Work out the finished part from the listing and answer in its coordinate system (mm). Face numbers are marked on the shaded views. Coordinates: 2 decimals unless noted, no trailing zeros. Order: outer loops, then holes, each group sorted by start corner. A loop starts at its lowest first (then second) coordinate and runs counter-clockwise, first axis right, second up. Notation, with made-up numbers: M -7,-29 L 15,-29 A31 cw 15,0 Z; hole C 80,17 d6. An arc over 180 degrees is marked long. Write item = value, one per line. Start each with the question number.
Q1. Find section C-C on y = 22. Give the vertices of the cut face in (x, z).
Q2. Each of these flat-tipped pins is pushed along its axis until it touches: P1, Ø3, axis at x = 4.5, y = 25.5, coming from the -Z side; P2, Ø3, axis at y = -21.5, z = -2, coming from the -X side; P3, Ø6, axis at x = 0, z = 0, coming from the +Y side. Where does it stop, or does it pass through?
Q3. Determine the mould class of the marked faces 1, 2 and 3 for opening direction Z: released by +Z, released by -Z, zero draft, split by the parting line, or undercut.
Q4. Find section D-D on x = 5.75. Give the vertices of the cut face in (y, z), and give its area (3 significant figures).
Q5. Find section A-A on z = 0. Give the vertices of the cut face in (x, y).
Q6. Straight lines are drawn through the part: line 1 along X through (y, z) = (38.8, 0); line 2 along X through (y, z) = (39.1, 0); line 3 along Y through (x, z) = (-3, 5.25). For each, find the intervals that lie inside material, in ascending order.
```python
from build123d import *

# Parameters (mm, degrees)
CROQUIS1_W                          = 7.5
CROQUIS1_H                          = 47.25
CROQUIS2_R                          = 3.2
SALIENTE_EXTRUIR1_DEPTH             = 1
CROQUIS3_R                          = 2.5
SALIENTE_EXTRUIR2_DEPTH             = 23
CORTAR_EXTRUIR1_START               = -20
CORTAR_EXTRUIR1_DEPTH               = 20
DI_METRO_DE_TALADRO_6_4_6_4_1_D     = 6.4
DI_METRO_DE_TALADRO_6_4_6_4_1_DEPTH = 1
CROQUIS7_W                          = 2.5
CROQUIS7_H                          = 0.75
CHAFL_N1_SIZE                       = 0.25


with BuildPart() as part:
    # Croquis1 → Revolución1 (revolve)
    with BuildSketch(Plane(origin=(0, 0, 0), x_dir=(-1, 0, 0), z_dir=(0, 0, -1)), mode=Mode.PRIVATE) as revoluci_n1_sk:
        with Locations((-3.75, 15.625)):
            Rectangle(CROQUIS1_W, CROQUIS1_H)
    revolve(revoluci_n1_sk.sketch.rotate(Axis((0, -8, 0), (0, 1, 0)), 270), axis=Axis((0, -8, 0), (0, 1, 0)))

    # Croquis2 → Saliente-Extruir1 (add)
    with BuildSketch(Plane.XZ.offset(8)):
        with Locations(Location((0, 0, 0), (0, 0, 270))):
            Circle(CROQUIS2_R)
    extrude(amount=SALIENTE_EXTRUIR1_DEPTH)

    # Croquis3 → Saliente-Extruir2 (add)
    with BuildSketch(Plane.XZ.offset(9)):
        with Locations(Location((0, 0, 0), (0, 0, 270))):
            Circle(CROQUIS3_R)
    extrude(amount=SALIENTE_EXTRUIR2_DEPTH)

    # Croquis4 → Cortar-Extruir1 (cut)
    with BuildSketch(Plane.XZ.offset(32).offset(CORTAR_EXTRUIR1_START)):
        with BuildLine():
            Line((-1.356465997, 2.1), (1.356465997, 2.1))
            ThreePointArc((1.356465997, 2.1), (0, 2.5), (-1.356465997, 2.1))
        make_face()
    extrude(amount=CORTAR_EXTRUIR1_DEPTH, mode=Mode.SUBTRACT)

    # Diámetro de taladro Ø6.4 (6.4)1
    with Locations(Plane(origin=(0, 39.25, 0), x_dir=(1, 0, 0), z_dir=(0, 1, 0))):
        with Locations((0, 0)):
            Hole(DI_METRO_DE_TALADRO_6_4_6_4_1_D / 2, depth=DI_METRO_DE_TALADRO_6_4_6_4_1_DEPTH)

    # Croquis7 → Revolución2 (revolve)
    with BuildSketch(Plane(origin=(0, 0, 0), x_dir=(-1, 0, 0), z_dir=(0, 0, -1)), mode=Mode.PRIVATE) as revoluci_n2_sk:
        with Locations((-1.25, 38.625)):
            Rectangle(CROQUIS7_W, CROQUIS7_H)
    revolve(revoluci_n2_sk.sketch.rotate(Axis((0, 38.25, 0), (0, 1, 0)), 270), axis=Axis((0, 38.25, 0), (0, 1, 0)))

    # Chaflán1
    chafl_n1_edges = [part.edges().sort_by_distance(p)[0] for p in [
        (0, -9, 3.2),
        (-2.397915762, -32, -0.707106781),
        (3.2, 38.25, 0),
        (0, 39, -2.5),
    ]]
    chamfer(chafl_n1_edges, length=CHAFL_N1_SIZE)


solid = part.part
```
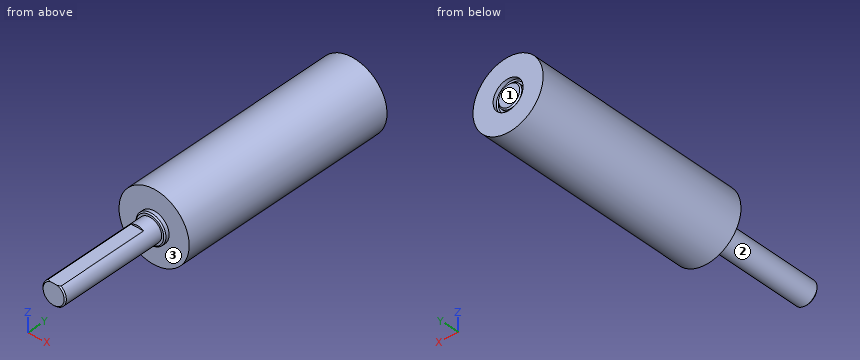
Findings below:
q1.outline = C 0,0 d15
q2.P1 = -6.87
q2.P2 = -2.45
q2.P3 = 39
q3.face_1 = undercut
q3.face_2 = split by the parting line
q3.face_3 = zero draft
q4.outline = M -8,-4.82 L 39.25,-4.82 L 39.25,4.82 L -8,4.82 Z
q4.area = 455 mm^2
q5.outline = M -7.5,-8 L -3.2,-8 L -3.2,-8.75 L -2.95,-9 L -2.5,-9 L -2.5,-31.75 L -2.25,-32 L 2.25,-32 L 2.5,-31.75 L 2.5,-9 L 2.95,-9 L 3.2,-8.75 L 3.2,-8 L 7.5,-8 L 7.5,39.25 L 3.2,39.25 L 3.2,38.5 L 2.95,38.25 L 2.5,38.25 L 2.5,38.75 L 2.25,39 L -2.25,39 L -2.5,38.75 L -2.5,38.25 L -2.95,38.25 L -3.2,38.5 L -3.2,39.25 L -7.5,39.25 Z
q6.line_1 = -7.5 to -3.2, -2.45 to 2.45, 3.2 to 7.5
q6.line_2 = -7.5 to -3.2, 3.2 to 7.5
q6.line_3 = -8 to 39.25
